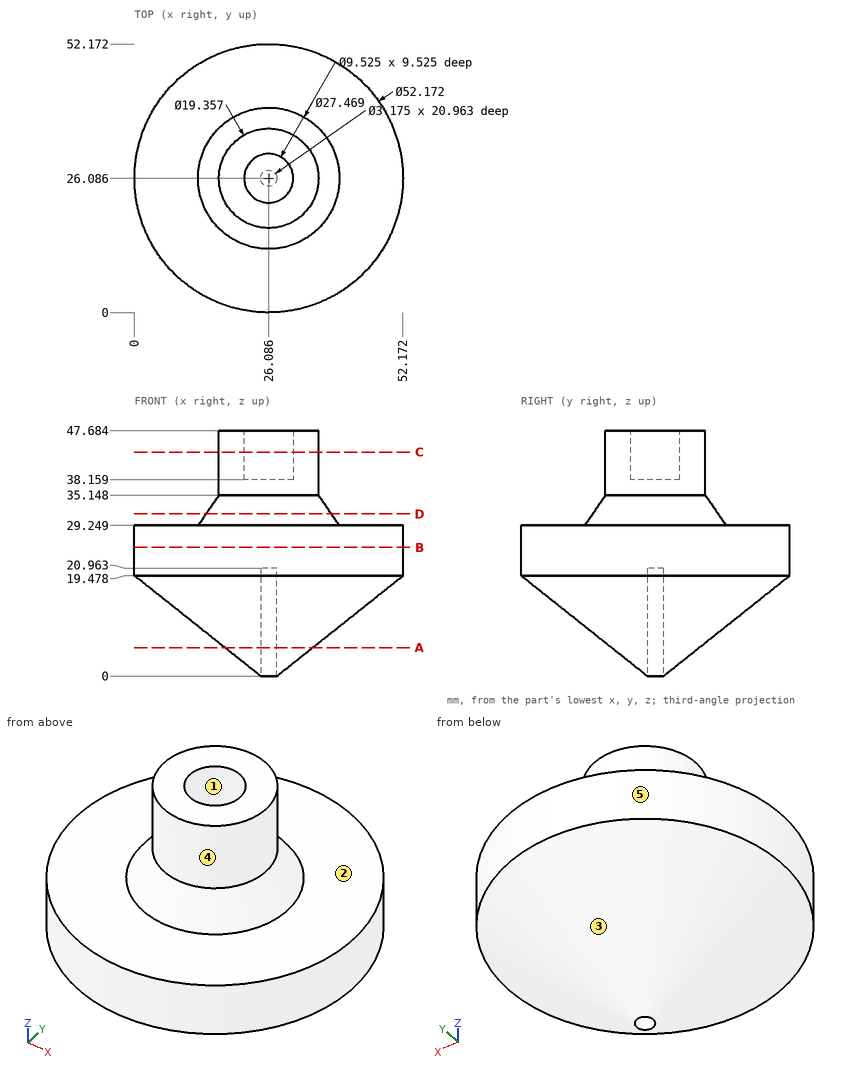
Geometry check sheet. Reference: drawing and pictorial views, mm from the part's lowest x, y, z. A direction names the side the tool comes from. Round coordinates to 2 decimals unless told otherwise and drop trailing zeros. Order: outer loops, then holes, each group sorted by start corner. A loop starts at its lowest first (then second) coordinate and runs counter-clockwise, first axis right, second up. Notation, with made-up numbers: (61, 65.25) - (73, 65.25) arc R35 cw to (73, 103.25) - close; hole circle Ø4 at (-26, 48). An arc over 180 degrees is marked (long way). Use a Markdown table: item, result. Add a question column.
1) Section check D-D (z = 31.5). Record the cut outline in (x, y), then the cut area to 3 significant figures.
2) Mould release check, pull along Y, two halves, no side actions. Record for the marked faces 1, 2 and 3: released by +Y, released by -Y, zero draft, split by the parting line, or undercut.
3) Section check C-C (z = 43.5). Record the cut outline in (x, y) (1 decimal), then the cut area to 3 significant figures.
4) Gauge pin test, flat ends, axial feed: P1, Ø8, axis at x = 7.5, y = 20.5, coming from the -Z side; P2, Ø12, axis at x = 17, y = 9, coming from the -Z side; P3, Ø4, axis at y = 10.5, z = 29, coming from the -X side. Record the tip position at first contact, or that the pin passes through.
5) Thickness scan on line 1 along X through (y, z) = (27, 21); line 2 along Z through (x, y) = (38.5, 21) (1 decimal); line 3 along X through (y, z) = (18.5, 8) (1 decimal). Record the ranges inside material, lowest first.
6) Section check B-B (z = 25). Record the cut outline in (x, y).
7) Set-up check for the marked faces 4 and 5: record each of +Z, -Z, +X, -X, +Y, -Y from which the full face is reachable in a straight line by a thin tool's end or side.
8) Section check A-A (z = 5.5). Record the cut outline in (x, y) (1 decimal), then the cut area to 3 significant figures.
Established:
| question | item | result |
|---|---|---|
| 1 | outline | circle Ø24.37 at (26.09, 26.09) |
| 1 | area | 467 mm2 |
| 2 | face 1 | undercut |
| 2 | face 2 | zero draft |
| 2 | face 3 | split by the parting line |
| 3 | outline | circle Ø19.4 at (26.1, 26.1); hole circle Ø9.5 at (26.1, 26.1) |
| 3 | area | 223 mm2 |
| 4 | P1 | z = 10.99 |
| 4 | P2 | z = 9.35 |
| 4 | P3 | x = 3.82 |
| 5 | line 1 | 0.02 to 52.16 |
| 5 | line 2 | 9.4 to 29.7 |
| 5 | line 3 | 17.2 to 34.9 |
| 6 | outline | circle Ø52.17 at (26.09, 26.09) |
| 7 | face 4 | +Z |
| 7 | face 5 | +Z, -Z |
| 8 | outline | circle Ø17 at (26.1, 26.1); hole circle Ø3.2 at (26.1, 26.1) |
| 8 | area | 219 mm2 |
